The model under review builds one solid part; all positions refer to its coordinate system, in mm. A direction names the side the tool comes from. Round coordinates to 2 decimals unless told otherwise and drop trailing zeros. Write each loop counter-clockwise with the first axis right and the second up, starting at its lowest first coordinate (ties: lowest second). Pieces come first, ordered by that corner, then holes. Notation, with made-up numbers: (57, 0) -> (90, 0) arc R17 cw to (90, 27) -> close; hole circle Ø2 at (60, -32.5). An arc over 180 degrees is marked (long way). Return JSON: item names as keys, results as strings. Group by question number.
1. Mouldability with a two-part tool opening along X and no side actions: class faces 3 (the flat face through (11, 0, 2)), 4 (the cylindrical face through (11.7, -3.6, 1.3)), 5 (the flat face through (40, -20, 1)), 6 (the cylindrical face through (37.2, -3.6, 1.3)) as pulls with the +X half, pulls with the -X half, needs draft (parallel to the pull), parting line crosses it, or undercut.
2. Take a section at B-B, the plane z = 20. Write out the cut boundary in (x, y).
3. Take a section at A-A, the plane x = 20. Write out the cut boundary in (y, z), then the cut area to 3 significant figures.
4. Clearance check with flat-ended pins moving along their axes: P1, Ø8, axis at y = -34.5, z = 32.5, coming from the +X side; P2, Ø6, axis at x = 12, y = -11.5, coming from the +Z side. State where each tip first meets the part, or that it passes through.
5. For line 1 along Y through (x, z) = (34, 1); line 2 along X through (y, z) = (-34, 1), list the stretches that pass through material, from the lowest coordinate up. Write a range as from..to.
6. Take a section at D-D, the plane x = 8.5. Write out the cut boundary in (y, z), then the cut area to 3 significant figures.
7. Take a section at C-C, the plane y = -34. Write out the cut boundary in (x, z), then the cut area to 3 significant figures.
8. Tool access review of faces 1 (the flat face through (25, -15, 2.5)), 2 (the cylindrical face through (1.3, -3.6, 5.3)): name each direction out of +Z, -Z, +X, -X, +Y, -Y from which nothing blocks a thin tool from reaching the whole face with its end or side.
from build123d import *

# Parameters (mm, degrees)
PAD_DEPTH       = 40
SKETCH001_R     = 4
POCKET_DEPTH    = 2.501
SKETCH002_R     = 4
SKETCH002_R_2   = 6
POCKET001_DEPTH = 2.501


with BuildPart() as part:
    # Sketch → Pad (new body)
    with BuildSketch(Plane.XZ):
        Polygon((0, 0), (0, 40), (2.5, 40), (2.5, 2.5), (40, 2.5), (40, 0), align=None)
    extrude(amount=PAD_DEPTH)

    # Sketch001 (on Face3 of Pad) → Pocket (cut, through all)
    with BuildSketch(Plane(origin=(2.5, 0, 0), x_dir=(0, 0, 1), z_dir=(1, 0, 0))):
        with Locations((8.5, 34)):
            Circle(SKETCH001_R)
        with Locations((34, 34)):
            Circle(SKETCH001_R)
        with Locations((8.5, 6)):
            Circle(SKETCH001_R)
        with Locations((34, 6)):
            Circle(SKETCH001_R)
        with Locations((20, 20)):
            Circle(SKETCH001_R)
    extrude(amount=-POCKET_DEPTH, mode=Mode.SUBTRACT)

    # Sketch002 (on Face13 of Pocket) → Pocket001 (cut, through all)
    with BuildSketch(Plane(origin=(0, 0, 2.5), x_dir=(-1, 0, 0), z_dir=(0, 0, 1))):
        with Locations((-8.5, 6)):
            Circle(SKETCH002_R)
        with Locations((-34, 6)):
            Circle(SKETCH002_R)
        with Locations((-8.5, 34)):
            Circle(SKETCH002_R)
        with Locations((-34, 34)):
            Circle(SKETCH002_R)
        with Locations((-20, 20)):
            Circle(SKETCH002_R_2)
    extrude(amount=-POCKET001_DEPTH, mode=Mode.SUBTRACT)


solid = part.part
Output:
{
 "1": {"face 3": "needs draft", "face 4": "undercut", "face 5": "pulls with the +X half", "face 6": "undercut"},
 "2": {"outline": "(0, -40) -> (2.5, -40) -> (2.5, -24) -> (0, -24) -> close; (0, -16) -> (2.5, -16) -> (2.5, 0) -> (0, 0) -> close"},
 "3": {"outline": "(-40, 0) -> (-26, 0) -> (-26, 2.5) -> (-40, 2.5) -> close; (-14, 0) -> (0, 0) -> (0, 2.5) -> (-14, 2.5) -> close", "area": "70.0 mm^2"},
 "4": {"P1": "stops at x = 2.5", "P2": "stops at z = 2.5"},
 "5": {"line 1": "y = -40..-38, -30..-10, -2..0", "line 2": "x = 0..4.5, 12.5..30, 38..40"},
 "6": {"outline": "(-40, 0) -> (-38, 0) -> (-38, 2.5) -> (-40, 2.5) -> close; (-30, 0) -> (-10, 0) -> (-10, 2.5) -> (-30, 2.5) -> close; (-2, 0) -> (0, 0) -> (0, 2.5) -> (-2, 2.5) -> close", "area": "60.0 mm^2"},
 "7": {"outline": "(0, 0) -> (4.5, 0) -> (4.5, 2.5) -> (2.5, 2.5) -> (2.5, 4.5) -> (0, 4.5) -> close; (0, 12.5) -> (2.5, 12.5) -> (2.5, 30) -> (0, 30) -> close; (0, 38) -> (2.5, 38) -> (2.5, 40) -> (0, 40) -> close; (12.5, 0) -> (30, 0) -> (30, 2.5) -> (12.5, 2.5) -> close; (38, 0) -> (40, 0) -> (40, 2.5) -> (38, 2.5) -> close", "area": "114 mm^2"},
 "8": {"face 1": "+Z, +X, +Y, -Y", "face 2": "+X, -X"}
}
